from build123d import *

# Parameters (mm, degrees)
HEXAGONALHEAD_DEPTH       = 5.25
SKETCH3_R                 = 2.5
CIRCULARCENTRALHOLE_DEPTH = 24


with BuildPart() as part:
    # Sketch1 → AluminiumPart (revolve)
    with BuildSketch(Plane.XY):
        Polygon((0, 4), (28.5, 4), (30.5, 2.5), (60.5, 2.5), (60.5, 0), (0, 0), align=None)
    revolve(axis=Axis((184.722030444, 0, 0), (-1, 0, 0)))

    # Sketch2 → HexagonalHead (cut)
    with BuildSketch(Plane.ZY):
        Polygon((-2.8, 1.616580754), (0, 3.233161507), (2.8, 1.616580754), (2.8, -1.616580754), (0, -3.233161507), (-2.8, -1.616580754), align=None)
    extrude(amount=-HEXAGONALHEAD_DEPTH, mode=Mode.SUBTRACT)

    # Sketch3 → CircularCentralHole (cut)
    with BuildSketch(Plane.ZY):
        Circle(SKETCH3_R)
    extrude(amount=-CIRCULARCENTRALHOLE_DEPTH, mode=Mode.SUBTRACT)

    # Sketch4 → FirstGreenPart (revolve)
    with BuildSketch(Plane.XY):
        Polygon((60.5, 0), (60.5, 2.5), (67.5, 5.5), (67.5, 0), align=None)
    revolve(axis=Axis((184.722030444, 0, 0), (-1, 0, 0)))

    # Sketch5 → FirstBlackPart (revolve)
    with BuildSketch(Plane.XY):
        with BuildLine():
            Line((67.5, 6.195683888), (77.5, 7.15))
            ThreePointArc((77.5, 7.15), (87, 7.602272753), (96.5, 7.15))
            Line((96.5, 7.15), (96.5, 0))
            Line((96.5, 0), (67.5, 0))
            Line((67.5, 0), (67.5, 6.195683888))
        make_face()
    revolve(axis=Axis((184.722030444, 0, 0), (-1, 0, 0)))

    # Sketch6 → SecondGreenPart (revolve)
    with BuildSketch(Plane.XY):
        with BuildLine():
            Line((152.5, 8), (152.5, 0))
            Line((152.5, 0), (96.5, 0))
            Line((96.5, 0), (96.5, 7.15))
            ThreePointArc((96.5, 7.15), (123.675746685, 6.231641521), (150.66986499, 9.5))
            ThreePointArc((150.66986499, 9.5), (151.939948886, 9.183151951), (152.5, 8))
        make_face()
    revolve(axis=Axis((184.722030444, 0, 0), (-1, 0, 0)))

    # Sketch7 → LastBlackPart (revolve)
    with BuildSketch(Plane.XY):
        with BuildLine():
            Line((152.5, 0), (152.5, 8))
            ThreePointArc((152.5, 8), (157.517257353, 6.700790451), (162.5, 8.126655981))
            ThreePointArc((162.5, 8.126655981), (163.829223328, 8.147753643), (164.5, 7))
            Line((164.5, 7), (164.5, 0))
            Line((164.5, 0), (152.5, 0))
        make_face()
    revolve(axis=Axis((184.722030444, 0, 0), (-1, 0, 0)))


solid = part.part
Design review of the part built by this model. Coordinates are the model's own, in mm. A direction names the side the tool comes from. Coordinates: 2 decimals unless noted, no trailing zeros. Order: outer loops, then holes, each group sorted by start corner. A loop starts at its lowest first (then second) coordinate and runs counter-clockwise, first axis right, second up. Notation, with made-up numbers: (19.5, 51.25) - (56.5, 51.25) arc R34 ccw to (56.5, 90.25) - close; hole circle Ø1 at (39.25, 47.25). An arc over 180 degrees is marked (long way). Put each result on its own line as item: value.
1) Insertion check: P1, Ø10, axis at x = 95.5, z = -4.5, coming from the +Y side; P2, Ø3, axis at x = 98, z = -1, coming from the -Y side (3 decimals); P3, Ø2, axis at x = 124, z = -4.5, coming from the -Y side; P4, Ø1, axis at x = 43.5, z = -4, coming from the -Y side. Each pin has a flat end and moves straight along its axis. Give the tip position at first contact, or say it passes through.
Response values:
P1: stops at y = 7.43
P2: stops at y = -7.125
P3: stops at y = -5.18
P4: passes through
2) Tool access review of faces 4 (the face through (14.45, -0.867, 3.905)), 5 (the face through (45.71, -0.54, 2.44)), 6 (the face through (0, 0, 3)): name each direction out of +Z, -Z, +X, -X, +Y, -Y from which nothing blocks a thin tool from reaching the whole face with its end or side.
Response values:
face 4: -X
face 5: none
face 6: +Z, -Z, -X, +Y, -Y
3) Take a section at B-B, the plane x = 63. Give the boundary of the cut face in (y, z).
Response values:
outline: circle Ø7.14 at (0, 0)
4) Take a section at A-A, the plane x = 40. Give the boundary of the cut face in (y, z), and give its area (3 significant figures).
Response values:
outline: circle Ø5 at (0, 0)
area: 19.6 mm²
5) The part is to be moulded in two halves that separate along X. For faces 1 (the face through (164.5, 0, 0)), 2 (the face through (3, 0, -2.8)), 3 (the face through (62.493, 3.199, -1.008)), say which applies: released by +X, released by -X, zero draft, split by the parting line, or undercut.
Response values:
face 1: released by +X
face 2: zero draft
face 3: undercut
6) Wall thickness on L1, parallel to Y at x = 15.25, z = 0; L2, parallel to Y at x = 78.5, z = -1.25; L3, parallel to X at y = 1.25, z = -0.25: over which ranges is each line inside the solid? List them lowest first. Write a range as from..to.
Response values:
L1: y = -4..-2.5, 2.5..4
L2: y = -7.13..7.13
L3: x = 24..164.5
